```python
from build123d import *

# Parameters (mm, degrees)
F0_W     = 31.75
F0_H     = 31.75
F1_DEPTH = 10.16
F2_R     = 2.54
F4_R     = 2.2606
F5_DEPTH = 25.4
F7_DEPTH = 3.81


with BuildPart() as f1:
    # F0 (on Top) → F1 (new body)
    with BuildSketch(Plane.XY):
        Rectangle(F0_W, F0_H)
    extrude(amount=F1_DEPTH)

    # F2 (on Front) → F3 (revolve, cut)
    with BuildSketch(Plane.XZ):
        with Locations((5.715, 10.16)):
            Circle(F2_R)
    revolve(axis=Axis((0, 0, 8.061379), (0, 0, -1)), mode=Mode.SUBTRACT)

    # F4 (on face) → F5 (cut)
    with BuildSketch(Plane.XY.offset(10.16)):
        Circle(F4_R)
        with Locations((-8.980256, 8.980256)):
            Circle(F4_R)
        with Locations((8.980256, 8.980256)):
            Circle(F4_R)
        with Locations((-8.980256, -8.980256)):
            Circle(F4_R)
        with Locations((8.980256, -8.980256)):
            Circle(F4_R)
    extrude(amount=-F5_DEPTH, mode=Mode.SUBTRACT)

    # F6 (on face) → F7 (cut)
    with BuildSketch(Plane(origin=(0, 0, 0), x_dir=(1, 0, 0), z_dir=(0, 0, -1))):
        Polygon((-2.4765, -4.289424), (2.4765, -4.289424), (4.953, 0), (2.4765, 4.289424), (-2.4765, 4.289424), (-4.953, 0), align=None)
        Polygon((-11.456756, 4.690832), (-6.503756, 4.690832), (-4.027256, 8.980256), (-6.503756, 13.26968), (-11.456756, 13.26968), (-13.933256, 8.980256), align=None)
        Polygon((11.456756, 13.26968), (6.503756, 13.26968), (4.027256, 8.980256), (6.503756, 4.690832), (11.456756, 4.690832), (13.933256, 8.980256), align=None)
        Polygon((4.027256, -8.980256), (6.503756, -13.26968), (11.456756, -13.26968), (13.933256, -8.980256), (11.456756, -4.690832), (6.503756, -4.690832), align=None)
        Polygon((-4.027256, -8.980256), (-6.503756, -4.690832), (-11.456756, -4.690832), (-13.933256, -8.980256), (-11.456756, -13.26968), (-6.503756, -13.26968), align=None)
    extrude(amount=-F7_DEPTH, mode=Mode.SUBTRACT)


solid = f1.part
```
Design review of the part built by this model. Coordinates are the model's own, in mm. A direction names the side the tool comes from. Coordinates: 2 decimals unless noted, no trailing zeros. Write each loop counter-clockwise with the first axis right and the second up, starting at its lowest first coordinate (ties: lowest second). Pieces come first, ordered by that corner, then holes.
1) Add section D-D (z = 9.75). Write out the cut boundary in (x, y) (3 decimals), plus the area to 3 significant figures.
2) Insertion check: pin 1 (1.5 mm diameter, centred on x = 9, y = 10, fed in from +Z). The pin has a flat end and moves straight along its axis. Give the tip position at first contact, or say it passes through.
3) Add section A-A (x = 0). Write out the cut boundary in (y, z) (3 decimals).
4) Machinability: for faces 1 (the flat face through (9, 13.27, 2)), 2 (the cylindrical face through (-0.49, -2.207, 7.029)), which of the approach directions +Z, -Z, +X, -X, +Y, -Y give a long, thin tool a straight path to every point of the face, cutting with its end or side? Answer none if there is none.
5) Add section B-B (z = 3). State how many separate pieces and enclosed holes the cut face has, plus the area to 3 significant figures.
6) Mouldability with a two-part tool opening along Y and no side actions: class faces 3 (the flat face through (5.248, 11.095, 1.878)), 4 (the flat face through (-7, 7, 10.16)), 5 (the flat face through (3.732, -2.115, 1.878)) as +Y half, -Y half, draft (parallel to the pull), parting line (faces both ways), or undercut.
7) To check wall thickness, follow L1, parallel to Y at x = -7.5, z = 1.5 (3 decimals); L2, parallel to X at y = 12.5, z = 2.75 (3 decimals); L3, parallel to X at y = -9.5, z = 5 (3 decimals). State the ranges of each line that lie inside material, in increasing order.
8) Add section C-C (y = -9.5). Write out the cut boundary in (x, z) (3 decimals).
Check result:
1. outline: (-15.875, -15.875) - (15.875, -15.875) - (15.875, 15.875) - (-15.875, 15.875) - close; circle Ø6.417 at (0, 0); hole circle Ø4.521 at (-8.98, -8.98); hole circle Ø4.521 at (-8.98, 8.98); hole circle Ø16.443 at (0, 0); hole circle Ø4.521 at (0, 0); hole circle Ø4.521 at (8.98, -8.98); hole circle Ø4.521 at (8.98, 8.98)
1. area: 748 mm2
2. pin 1: passes through
3. outline: (-15.875, 0) - (-4.289, 0) - (-4.289, 3.81) - (-2.261, 3.81) - (-2.261, 10.16) - (-3.175, 10.16) arc R2.54 cw to (-8.255, 10.16) - (-15.875, 10.16) - close; (2.261, 3.81) - (4.289, 3.81) - (4.289, 0) - (15.875, 0) - (15.875, 10.16) - (8.255, 10.16) arc R2.54 cw to (3.175, 10.16) - (2.261, 10.16) - close
4. face 1: -Z
4. face 2: +Z, -Z
5. separate pieces: 1
5. enclosed holes: 5
5. area: 689 mm2
6. face 3: undercut
6. face 4: draft
6. face 5: undercut
7. L1: y = -15.875 to -13.27, -4.691 to 4.691, 13.27 to 15.875
7. L2: x = -15.875 to -11.901, -6.059 to 6.059, 11.901 to 15.875
7. L3: x = -15.875 to -11.18, -6.78 to 6.78, 11.18 to 15.875
8. outline: (-15.875, 0) - (-13.633, 0) - (-13.633, 3.81) - (-11.18, 3.81) - (-11.18, 10.16) - (-15.875, 10.16) - close; (-6.78, 3.81) - (-4.327, 3.81) - (-4.327, 0) - (4.327, 0) - (4.327, 3.81) - (6.78, 3.81) - (6.78, 10.16) - (-6.78, 10.16) - close; (11.18, 3.81) - (13.633, 3.81) - (13.633, 0) - (15.875, 0) - (15.875, 10.16) - (11.18, 10.16) - close
